```python
from build123d import *

# Parameters (mm, degrees)
SKETCH1_W           = 1.7
SKETCH1_H           = 16
BOSS_EXTRUDE1_DEPTH = 10


with BuildPart() as part:
    # Sketch1 → Boss-Extrude1 (new body)
    with BuildSketch(Plane.XY):
        with BuildLine():
            Line((8.5, -13), (9.5, -13))
            Line((9.5, -13), (9.5, -15))
            Line((9.5, -15), (7.5, -15))
            Line((7.5, -15), (7.5, -16.5))
            Line((7.5, -16.5), (13.104700538, -16.5))
            Line((13.104700538, -16.5), (11.95, -14.5))
            Line((11.95, -14.5), (11.95, 9))
            ThreePointArc((11.95, 9), (-3.764514939, 10.079270346), (-11.95, -3.378390615))
            Line((-11.95, -3.378390615), (-11.95, -14.5))
            Line((-11.95, -14.5), (-13.104700538, -16.5))
            Line((-13.104700538, -16.5), (-7.5, -16.5))
            Line((-7.5, -16.5), (-7.5, -15))
            Line((-7.5, -15), (-9.5, -15))
            Line((-9.5, -15), (-9.5, -13))
            Line((-9.5, -13), (-8.5, -13))
            Line((-8.5, -13), (-8.5, -11.5))
            Line((-8.5, -11.5), (-10.5, -11.5))
            Line((-10.5, -11.5), (-10.5, -10))
            Line((-10.5, -10), (-7, -10))
            Line((-7, -10), (-7, -4.366062299))
            ThreePointArc((-7, -4.366062299), (0, 8.25), (7, -4.366062299))
            Line((7, -4.366062299), (7, -10))
            Line((7, -10), (10.5, -10))
            Line((10.5, -10), (10.5, -11.5))
            Line((10.5, -11.5), (8.5, -11.5))
            Line((8.5, -11.5), (8.5, -13))
        make_face()
        with Locations((10.1, -0.5)):
            Rectangle(SKETCH1_W, SKETCH1_H, mode=Mode.SUBTRACT)
    extrude(amount=BOSS_EXTRUDE1_DEPTH)


solid = part.part
```
Here's how the part is built. I have some questions about the finished solid (model axes, mm). A direction names the side the tool comes from. Give positions to 0.01 mm unless a question says otherwise; leave off trailing zeros. Write each loop counter-clockwise with the first axis right and the second up, starting at its lowest first coordinate (ties: lowest second). Pieces come first, ordered by that corner, then holes.
(1) On a 3-axis mill with a long thin cutter (end or side, diameter ignored), from which of +Z, -Z, +X, -X, +Y, -Y can I reach the whole of each face in a straight line? I mean faces 1 (the face through (7.5, -16, 5)), 2 (the face through (-9, -11.5, 5)), 3 (the face through (11.95, -3, 5)). Say none if no direction works.
Output values:
face 1: +Z, -Z, -Y
face 2: +Z, -Z
face 3: +Z, -Z, +X, +Y
(2) Imagine slicing it at D-D, the plane y = 0. Write out the boundary of the cut face in (x, z).
Output values:
outline: (-11.57, 0) - (-8.25, 0) - (-8.25, 10) - (-11.57, 10) - close; (8.25, 0) - (9.25, 0) - (9.25, 10) - (8.25, 10) - close; (10.95, 0) - (11.95, 0) - (11.95, 10) - (10.95, 10) - close
(3) If I drill on L1, parallel to X at y = -5, z = 6.25; L2, parallel to X at y = 0, z = 5.25; L3, parallel to X at y = -13.25, z = 3.75, over which ranges is the centre line in solid material (lowest first)?
Output values:
L1: x = -11.95 to -7, 7 to 9.25, 10.95 to 11.95
L2: x = -11.57 to -8.25, 8.25 to 9.25, 10.95 to 11.95
L3: x = -11.95 to -9.5, 9.5 to 11.95
(4) Imagine slicing it at A-A, the plane y = -5. Write out the boundary of the cut face in (x, z).
Output values:
outline: (-11.95, 0) - (-7, 0) - (-7, 10) - (-11.95, 10) - close; (7, 0) - (9.25, 0) - (9.25, 10) - (7, 10) - close; (10.95, 0) - (11.95, 0) - (11.95, 10) - (10.95, 10) - close
(5) Will these pins go through, and if not, where does the flat tip stop? pin 1 (5 mm diameter, centred on y = 3.5, z = 6.5, fed in from -X); pin 2 (0.8 mm diameter, centred on y = -12, z = 5.5, fed in from -X); pin 3 (0.8 mm diameter, centred on x = 10, z = 5.5, fed in from +Y).
Output values:
pin 1: stops at x = -11.3
pin 2: stops at x = -11.95
pin 3: stops at y = 10.36
(6) Imagine slicing it at C-C, the plane x = -1. Write out the boundary of the cut face in (y, z), and give its area (3 significant figures).
Output values:
outline: (8.19, 0) - (11.18, 0) - (11.18, 10) - (8.19, 10) - close
area: 29.9 mm2
(7) Thinking about a two-plate mould opening in X: for faces 4 (the face through (12.535, -15.514, 4.93)), 5 (the face through (-10, -16.5, 5)), 6 (the face through (10, -8.5, 5)), which applies, pulls with the +X half, pulls with the -X half, needs draft (parallel to the pull), parting line crosses it, or undercut?
Output values:
face 4: pulls with the +X half
face 5: needs draft
face 6: undercut
